Autodesk Inventor part; units mm, degrees
ref_plane "YZ Plane" through (0, 0, 0) normal (1, 0, 0) x (0, 1, 0)
ref_plane "XZ Plane" through (0, 0, 0) normal (0, 1, 0) x (-1, 0, 0)
ref_plane "XY Plane" through (0, 0, 0) normal (0, 0, 1) x (1, 0, 0)
sketch "草圖1" plane through (0, 0, 0) normal (0, 1, 0) x (-1, 0, 0)
  circle A0 centre (0, 0) radius 12.5
  circle A1 centre (0, 8.5) radius 1.5
  circle A2 centre (0, -8.5) radius 1.5
  dimension "d0" = 25
  dimension "d1" = 17
  dimension "d2" = 8.5
  dimension "d3" = 3
  dimension "d4" = 3
extrude "擠出1" add sketch "草圖1" along normal blind 6
sketch "草圖2" plane through (0, 6, 0) normal (0, 1, 0) x (1, 0, 0)
  circle A0 centre (0, 0) radius 5.5
  dimension "d7" = 11
extrude "擠出2" cut sketch "草圖2" against normal through all
sketch "草圖3" plane through (0, 6, 0) normal (0, 1, 0) x (1, 0, 0)
  circle A0 centre (0, 0) radius 6.5
  dimension "d10" = 13
extrude "擠出3" cut sketch "草圖3" against normal blind 5
move faces "移動1" translate (0, -1.25, 0) faces at (3.8939, 0, -7.6516)
properties part number "wheel_base_cover"
Geometry check sheet. Reference: the model listing, model coordinates, mm. A direction names the side the tool comes from. Round coordinates to 2 decimals unless told otherwise and drop trailing zeros. Write each loop counter-clockwise with the first axis right and the second up, starting at its lowest first coordinate (ties: lowest second). Pieces come first, ordered by that corner, then holes. Notation, with made-up numbers: (-23.75, 36) - (8.25, 36) arc R20 ccw to (8.25, 40) - close; hole circle Ø1 at (89.5, 57). An arc over 180 degrees is marked (long way). One line per item, written item: value.
1. Cross-section at C-C on x = -4.75. Record the boundary of the cut face in (y, z).
The answers:
outline: (-1.25, -11.56) - (6, -11.56) - (6, -4.44) - (1, -4.44) - (1, -2.77) - (-1.25, -2.77) - close; (-1.25, 2.77) - (1, 2.77) - (1, 4.44) - (6, 4.44) - (6, 11.56) - (-1.25, 11.56) - close
2. Scan lines: L1, parallel to Z at x = 0, y = 2; L2, parallel to Z at x = 0, y = -0.1; L3, parallel to X at y = -0.6, z = 0. Record each from-to range of solid material in increasing order.
The answers:
L1: z = -12.5 to -10, -7 to -6.5, 6.5 to 7, 10 to 12.5
L2: z = -12.5 to -10, -7 to -5.5, 5.5 to 7, 10 to 12.5
L3: x = -12.5 to -5.5, 5.5 to 12.5
3. Cross-section at A-A on x = 0. Record the boundary of the cut face in (y, z).
The answers:
outline: (-1.25, -12.5) - (6, -12.5) - (6, -10) - (-1.25, -10) - close; (-1.25, -7) - (6, -7) - (6, -6.5) - (1, -6.5) - (1, -5.5) - (-1.25, -5.5) - close; (-1.25, 5.5) - (1, 5.5) - (1, 6.5) - (6, 6.5) - (6, 7) - (-1.25, 7) - close; (-1.25, 10) - (6, 10) - (6, 12.5) - (-1.25, 12.5) - close
4. Depth check by flat-ended pin: pin 1 Ø2 at (x, y) = (5, 2) entering from -Z; pin 2 Ø4 at (x, z) = (-2, -1.5) entering from +Y; pin 3 Ø3 at (x, y) = (-9.5, 4) entering from -Z; pin 4 Ø1 at (y, z) = (0.5, 3) entering from -X. Enter the tip coordinate at first touch or a pass-through.
The answers:
pin 1: stops at z = -11.84
pin 2: passes through
pin 3: stops at z = -9.6
pin 4: stops at x = -12.25
5. Set-up check for faces 1 (the face through (-5, 6, -5)), 2 (the face through (-5.158, 3.535, 3.955)): record each of +Z, -Z, +X, -X, +Y, -Y from which the full face is reachable in a straight line by a thin tool's end or side.
The answers:
face 1: +Z, -Z, +X, -X, +Y
face 2: +Y
6. Cross-section at D-D on y = 5. Record the boundary of the cut face in (x, z).
The answers:
outline: circle Ø25 at (0, 0); hole circle Ø13 at (0, 0); hole circle Ø3 at (0, -8.5); hole circle Ø3 at (0, 8.5)
7. Mould release check, pull along X, two halves, no side actions. Record for faces 3 (the face through (-11.923, 2.324, -3.755)), 4 (the face through (-3, -1.25, -5)), 5 (the face through (-1.19, -0.11, 5.37)): released by +X, released by -X, zero draft, split by the parting line, or undercut.
The answers:
face 3: split by the parting line
face 4: zero draft
face 5: undercut
8. Cross-section at B-B on z = 0. Record the boundary of the cut face in (x, y).
The answers:
outline: (-12.5, -1.25) - (-5.5, -1.25) - (-5.5, 1) - (-6.5, 1) - (-6.5, 6) - (-12.5, 6) - close; (5.5, -1.25) - (12.5, -1.25) - (12.5, 6) - (6.5, 6) - (6.5, 1) - (5.5, 1) - close
